Model file for the job. Use its own axes, mm. A direction names the side the tool comes from. Give positions to 0.01 mm unless a question says otherwise; leave off trailing zeros. Order: outer loops, then holes, each group sorted by start corner. A loop starts at its lowest first (then second) coordinate and runs counter-clockwise, first axis right, second up. Notation, with made-up numbers: (27.25, 82) - (48.25, 82) arc R28 cw to (48.25, 108) - close; hole circle Ø6 at (85.5, 60). An arc over 180 degrees is marked (long way). Return JSON: item names as keys, results as strings. Group by question number.
from build123d import *

# Parameters (mm, degrees)
F0_R          = 8.25
F0_R_2        = 6.25
F1_DEPTH      = 40
F2_W          = 20.5353749644
F2_H          = 10
F2_R          = 1
F3_DEPTH      = 25
F3_DEPTH_BACK = 25
F4_R          = 1
F4_W          = 9.5603424124
F4_H          = 10
F5_DEPTH      = 25
F5_DEPTH_BACK = 25


with BuildPart() as f1:
    # F0 (on Right) → F1 (new body)
    with BuildSketch(Plane.YZ):
        Circle(F0_R)
        Circle(F0_R_2, mode=Mode.SUBTRACT)
    extrude(amount=F1_DEPTH)

    # F2 (on Top) → F3 (cut, two sides)
    with BuildSketch(Plane.XY) as f3_sk:
        with Locations((42.2676874822, 0)):
            Rectangle(F2_W, F2_H)
        with Locations((3, 0)):
            Circle(F2_R)
    extrude(amount=-F3_DEPTH, mode=Mode.SUBTRACT)
    extrude(f3_sk.sketch, amount=F3_DEPTH_BACK, mode=Mode.SUBTRACT)

    # F4 (on Front) → F5 (cut, two sides)
    with BuildSketch(Plane.XZ) as f5_sk:
        with Locations((37, 0)):
            Circle(F4_R)
        with Locations((3.2198287938, 0)):
            Rectangle(F4_W, F4_H)
    extrude(amount=-F5_DEPTH, mode=Mode.SUBTRACT)
    extrude(f5_sk.sketch, amount=F5_DEPTH_BACK, mode=Mode.SUBTRACT)


solid = f1.part
(1) Drop flat-ended pins along their axis: pin 1 Ø0.8 at (x, z) = (34.5, -5.5) entering from -Y; pin 2 Ø0.8 at (x, y) = (5.5, 5.5) entering from +Z; pin 3 Ø1.4 at (x, y) = (5, -4.5) entering from -Z; pin 4 Ø8 at (y, z) = (-2.5, -1) entering from +X. Give the stop position or say it passes through.
(2) Slice it at A-A (y = 0). Give the cut face in (x, z).
(3) Slice it at D-D (z = 0). Give the cut face in (x, y).
(4) Pull direction Z, two halves, no side cores. Call faces 4 (the face through (36, -5, 5)), 5 (the face through (4, -5, -5)): released by +Z, released by -Z, zero draft, split by the parting line, or undercut.
(5) Slice it at B-B (x = 34). Give the cut face in (y, z), and give its area (3 significant figures).
(6) 3-axis set-ups, long thin cutter, end or side, ignore diameter. For faces 1 (the face through (32, -0.1, 6.5)), 2 (the face through (8, -6.5, -0.1)), 3 (the face through (0, 0, 7)): which of +Z, -Z, +X, -X, +Y, -Y reach the whole face in a straight line?
(7) Slice it at C-C (z = -2.75). Give the cut face in (x, y), and give its area (3 significant figures).
(8) Drill centre lines: L1, parallel to Y at x = 8.5, z = 5; L2, parallel to Z at x = 26, y = 0; L3, parallel to Z at x = 37, y = 7.05. Where is each one in solid material? Low to high.
Result set:
{
 "1": {"pin 1": "stops at y = -6.48", "pin 2": "stops at z = 6.48", "pin 3": "stops at z = -7.32", "pin 4": "stops at x = 40"},
 "2": {"outline": "(0, -8.25) - (2, -8.25) - (2, -6.25) - (0, -6.25) - close; (0, 6.25) - (2, 6.25) - (2, 8.25) - (0, 8.25) - close; (4, -8.25) - (32, -8.25) - (32, -6.25) - (4, -6.25) - close; (4, 6.25) - (32, 6.25) - (32, 8.25) - (4, 8.25) - close"},
 "3": {"outline": "(8, -8.25) - (36, -8.25) - (36, -6.25) - (8, -6.25) - close; (8, 6.25) - (36, 6.25) - (36, 8.25) - (8, 8.25) - close; (38, -8.25) - (40, -8.25) - (40, -6.25) - (38, -6.25) - close; (38, 6.25) - (40, 6.25) - (40, 8.25) - (38, 8.25) - close"},
 "4": {"face 4": "zero draft", "face 5": "undercut"},
 "5": {"outline": "(-5, -6.56) - (-5, -3.75) arc R6.25 cw to (-5, 3.75) - (-5, 6.56) arc R8.25 ccw to start; (5, -6.56) arc R8.25 ccw to (5, 6.56) - (5, 3.75) arc R6.25 cw to (5, -3.75) - close", "area": "46.8 mm²"},
 "6": {"face 1": "+Z, -Z, +X", "face 2": "-X, +Y, -Y", "face 3": "+Z, -Z, -X, +Y, -Y"},
 "7": {"outline": "(8, -7.78) - (40, -7.78) - (40, -5.61) - (8, -5.61) - close; (8, 5.61) - (40, 5.61) - (40, 7.78) - (8, 7.78) - close", "area": "139 mm²"},
 "8": {"L1": "y = -6.56 to -3.75, 3.75 to 6.56", "L2": "z = -8.25 to -6.25, 6.25 to 8.25", "L3": "z = -4.28 to -1, 1 to 4.28"}
}
